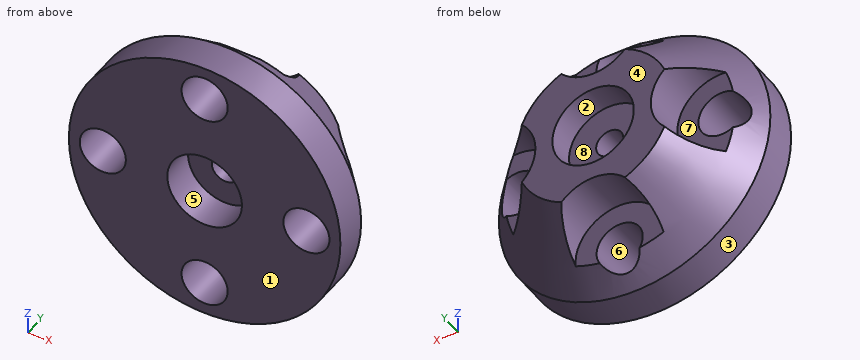
Autodesk Inventor part; units mm, degrees
ref_plane "YZ Plane" through (0, 0, 0) normal (1, 0, 0) x (0, 1, 0)
ref_plane "XZ Plane" through (0, 0, 0) normal (0, 1, 0) x (-1, 0, 0)
ref_plane "XY Plane" through (0, 0, 0) normal (0, 0, 1) x (1, 0, 0)
sketch "Sketch2" plane through (0, 0, 0) normal (0, 0, 1) x (1, 0, 0)
  line L0 (1, 2.5) -> (1, 5.5)
  line L1 (1, 5.5) -> (3, 5.5)
  line L2 (3, 5.5) -> (3, 7.5)
  line L3 (3, 7.5) -> (5.75, 7.5)
  line L4 (5.75, 7.5) -> (10, 2.5)
  line L5 (10, 2.5) -> (10, 0)
  line L6 (1, 2.5) -> (2.75, 2.5)
  line L7 (2.75, 2.5) -> (2.75, 0)
  line L8 (2.75, 0) -> (10, 0)
  line L9 (0, 0) -> (0, 19.425)
  dimension "d0" = 6
  dimension "d1" = 2
  dimension "d2" = 5.5
  dimension "d3" = 20
  dimension "d4" = 2.5
  dimension "d5" = 3
  dimension "d6" = 2
  dimension "d19" = 11.5
revolve "Revolution1" add sketch "Sketch2" angle 360 about axis through (0, 0, 0) along (0, 1, 0)
sketch "Sketch3" plane through (0, 7.5, 0) normal (0, 1, 0) x (1, 0, 0)
  point P0 (0, 0)
  point P1 (0, 7.5)
  dimension "d8" = 7.5
hole "Hole1" at (0, 7.5, -7.5) direction (0, -1, 0) diameter 3.4 end through all counterbore diameter 6.5 counterbore depth 3.2
pattern_circular "Circular Pattern1" count 4 over 360 about axis through (0, -10, 0) along (0, 1, 0) of "Hole1"
properties part number "902-4250 magnet hold"
Check sheet for the modelled part. Datum: model origin and axes. Units: mm. Face numbers are marked on the shaded views. A direction names the side the tool comes from. Coordinates: 2 decimals unless noted, no trailing zeros. Write each loop counter-clockwise with the first axis right and the second up, starting at its lowest first coordinate (ties: lowest second). Pieces come first, ordered by that corner, then holes. Notation, with made-up numbers: M 88,74 L 140,74 A25 cw 140,94 Z; hole C 38,7 d6. An arc over 180 degrees is marked long. Write item = value, one per line. Start each with the question number.
1. Tool access check on the marked faces 4, 5, 6, 7 and 8. Record the directions out of +Z, -Z, +X, -X, +Y, -Y that give a thin tool (end or side, any length) a straight path to the whole face; none if there is none.
2. Mould release check, pull along X, two halves, no side actions. Record for the marked faces 1, 2 and 3: pulls with the +X half, pulls with the -X half, needs draft (parallel to the pull), parting line crosses it, or undercut.
3. Sectioned sample at C-C (z = 0). Record the cut outline in (x, y), then the cut area to 3 significant figures.
4. Go/stop test with flat-tipped pins: pin 1 (12 mm diameter, centred on x = 5.5, z = 3.5, fed in from +Y); pin 2 (3.5 mm diameter, centred on x = 0, z = 0, fed in from -Y); pin 3 (3 mm diameter, centred on x = -6, y = 3, fed in from -Z); pin 4 (4 mm diameter, centred on x = 2, y = 6, fed in from -Z). Record where each tip stops, or that it passes through.
5. Sectioned sample at B-B (x = 0). Record the cut outline in (y, z), then the cut area to 3 significant figures.
6. Sectioned sample at A-A (y = 1). Record the cut outline in (x, z).
7. Thickness scan on probe 1 along Z at (x, y) = (0, 0.7); probe 2 along Z at (x, y) = (-8.25, 1.75); probe 3 along Y at (x, z) = (0.5, -4.5). Record the ranges inside material, lowest first.
8. Sectioned sample at D-D (y = 4). Record the cut outline in (x, z) (3 decimals).
The answers:
q1.face_4 = +Z, -Z, +X, -X, +Y
q1.face_5 = -Y
q1.face_6 = +Y, -Y
q1.face_7 = -X, +Y
q1.face_8 = +Y
q2.face_1 = needs draft
q2.face_2 = undercut
q2.face_3 = parting line crosses it
q3.outline = M -10,0 L -9.2,0 L -9.2,3.44 L -10,2.5 Z; M -5.8,0 L -2.75,0 L -2.75,2.5 L -1,2.5 L -1,5.5 L -3,5.5 L -3,7.5 L -4.25,7.5 L -4.25,4.3 L -5.8,4.3 Z; M 1,2.5 L 2.75,2.5 L 2.75,0 L 5.8,0 L 5.8,4.3 L 4.25,4.3 L 4.25,7.5 L 3,7.5 L 3,5.5 L 1,5.5 Z; M 9.2,0 L 10,0 L 10,2.5 L 9.2,3.44 Z
q3.area = 50.1 mm²
q4.pin_1 = 7.5
q4.pin_2 = 2.5
q4.pin_3 = -8.89
q4.pin_4 = -8.54
q5.outline = M 0,-10 L 2.5,-10 L 3.44,-9.2 L 0,-9.2 Z; M 0,-5.8 L 4.3,-5.8 L 4.3,-4.25 L 7.5,-4.25 L 7.5,-3 L 5.5,-3 L 5.5,-1 L 2.5,-1 L 2.5,-2.75 L 0,-2.75 Z; M 0,2.75 L 2.5,2.75 L 2.5,1 L 5.5,1 L 5.5,3 L 7.5,3 L 7.5,4.25 L 4.3,4.25 L 4.3,5.8 L 0,5.8 Z; M 0,9.2 L 3.44,9.2 L 2.5,10 L 0,10 Z
q5.area = 50.1 mm²
q6.outline = C 0,0 d20; hole C -7.5,0 d3.4; hole C 0,0 d5.5; hole C 0,-7.5 d3.4; hole C 0,7.5 d3.4; hole C 7.5,0 d3.4
q7.probe_1 = -10 to -9.2, -5.8 to -2.75, 2.75 to 5.8, 9.2 to 10
q7.probe_2 = -5.65 to -1.53, 1.53 to 5.65
q7.probe_3 = 0 to 4.3
q8.outline = M -8.632,-1.268 A8.725 ccw -1.268,-8.632 A1.7 cw long 1.268,-8.632 A8.725 ccw 8.632,-1.268 A1.7 cw long 8.632,1.268 A8.725 ccw 1.268,8.632 A1.7 cw long -1.268,8.632 A8.725 ccw -8.632,1.268 A1.7 cw long Z; hole C 0,0 d2
